```python
from build123d import *

# Parameters (mm, degrees)
SKETCH_1_R      = 17.5
SKETCH_1_R_2    = 12.5
EXTRUDE_1_DEPTH = 4


with BuildPart() as part:
    # 草图1 → 凸台-拉伸1 (new body)
    with BuildSketch(Plane.XY):
        with BuildLine():
            Line((-26.716521465, 615.290207127), (-146.53444515, 615.290207127))
            Line((-146.53444515, 615.290207127), (-156.716521465, 640.290207127))
            Line((-156.716521465, 640.290207127), (-156.716521465, 760.290207127))
            Line((-156.716521465, 760.290207127), (-33.233977794, 675.622063649))
            ThreePointArc((-33.233977794, 675.622063649), (-28.445535159, 670.242358457), (-26.716521465, 663.250869168))
            Line((-26.716521465, 663.250869168), (-26.716521465, 615.290207127))
        make_face()
        with Locations((-123.214216797, 685.589410404)):
            Circle(SKETCH_1_R, mode=Mode.SUBTRACT)
        with Locations((-71.258091401, 666.840828083)):
            Circle(SKETCH_1_R_2, mode=Mode.SUBTRACT)
    extrude(amount=EXTRUDE_1_DEPTH)


solid = part.part
```
Work out the finished part from the listing and answer in its coordinate system (mm). Give positions to 0.01 mm unless a question says otherwise; leave off trailing zeros. Loops run counter-clockwise (first coordinate to the right, second up) from the corner with the lowest first, then second, coordinate; pieces in that order, holes last. Notation, with made-up numbers: (17, 2) -> (73, 2) arc R34 ccw to (73, 41) -> close; hole circle Ø11 at (46, 37). An arc over 180 degrees is marked (long way). One line per question, with ' | ' between items. Start each with the question number.
1) Straight lines are drawn through the part: L1, parallel to X at y = 695, z = 3.65; L2, parallel to Y at x = -79.5, z = 2; L3, parallel to Y at x = -116, z = 0.7. For each, find the intervals that lie inside material, in ascending order.
2) Section D-D, the plane y = 627 is taken. Determine the outline of the cut face in (x, z), then the cut area to 3 significant figures.
3) Determine the mould class of faces 1 (the face through (-28.49, 670.33, 1.97)), 2 (the face through (-59.711, 662.053, 1.972)), 3 (the face through (-26.717, 640, 2)) for opening direction Y: +Y half, -Y half, draft (parallel to the pull), parting line (faces both ways), or undercut.
4) Section B-B, the plane y = 659.5 is taken. Determine the outline of the cut face in (x, z), then the cut area to 3 significant figures.
5) This flat-tipped pin is pushed along its axis until it touches: pin 1 (1 mm diameter, centred on y = 691, z = 2.5, fed in from +X). Where does it stop, or does it pass through?
6) Section C-C, the plane z = 1.4 is taken. Determine the outline of the cut face in (x, y).
7) Section A-A, the plane x = -68 is taken. Determine the outline of the cut face in (y, z), then the cut area to 3 significant figures.
Resolved:
1) L1: -156.72 to -137.97, -108.46 to -61.5 | L2: 615.29 to 657.44, 676.24 to 707.35 | L3: 615.29 to 669.65, 701.53 to 732.37
2) outline: (-151.3, 0) -> (-26.72, 0) -> (-26.72, 4) -> (-151.3, 4) -> close | area: 498 mm2
3) face 1: +Y half | face 2: undercut | face 3: draft
4) outline: (-156.72, 0) -> (-81.38, 0) -> (-81.38, 4) -> (-156.72, 4) -> close; (-61.14, 0) -> (-26.72, 0) -> (-26.72, 4) -> (-61.14, 4) -> close | area: 439 mm2
5) pin 1: x = -54.93
6) outline: (-156.72, 640.29) -> (-146.53, 615.29) -> (-26.72, 615.29) -> (-26.72, 663.25) arc R15 ccw to (-33.23, 675.62) -> (-156.72, 760.29) -> close; hole circle Ø35 at (-123.21, 685.59); hole circle Ø25 at (-71.26, 666.84)
7) outline: (615.29, 0) -> (654.77, 0) -> (654.77, 4) -> (615.29, 4) -> close; (678.91, 0) -> (699.46, 0) -> (699.46, 4) -> (678.91, 4) -> close | area: 240 mm2
